```python
from build123d import *

# Parameters (mm, degrees)
F0_R     = 57
F1_DEPTH = 5
F0_W     = 15
F0_H     = 15
F2_DEPTH = 20
F3_SIZE  = 5


with BuildPart() as f1:
    # F0 (on Top) → F1 (new body)
    with BuildSketch(Plane.XY):
        Polygon((-45, -60), (45, -60), (45, -45), (60, -45), (60, 45), (45, 45), (45, 60), (-45, 60), (-45, 45), (-60, 45), (-60, -45), (-45, -45), align=None)
        Circle(F0_R, mode=Mode.SUBTRACT)
    extrude(amount=F1_DEPTH)

    # F0 (on Top) → F2 (join)
    with BuildSketch(Plane.XY):
        with Locations((-52.5, 52.5)):
            Rectangle(F0_W, F0_H)
        with Locations((52.5, 52.5)):
            Rectangle(F0_W, F0_H)
        with Locations((52.5, -52.5)):
            Rectangle(F0_W, F0_H)
        with Locations((-52.5, -52.5)):
            Rectangle(F0_W, F0_H)
    extrude(amount=F2_DEPTH)

    # F3
    f3_edges = [f1.edges().sort_by_distance(p)[0] for p in [
        (-60, -45, 12.5),
        (-45, -60, 12.5),
        (45, -60, 12.5),
        (60, -45, 12.5),
        (45, 60, 12.5),
        (60, 45, 12.5),
        (-60, 45, 12.5),
        (-45, 60, 12.5),
    ]]
    chamfer(f3_edges, length=F3_SIZE)


solid = f1.part
```
CAD build for the part. Positions are in the model's coordinates, mm. A direction names the side the tool comes from. Coordinates: 2 decimals unless noted, no trailing zeros. Write each loop counter-clockwise with the first axis right and the second up, starting at its lowest first coordinate (ties: lowest second). Pieces come first, ordered by that corner, then holes. Notation, with made-up numbers: (83, 58) -> (118, 58) arc R9 cw to (118, 66) -> close; hole circle Ø3 at (40.25, -34.5). An arc over 180 degrees is marked (long way). Use CSV: the item, a comma, the result in double quotes. Start each with the question number.
Item 1: Two-plate mould, pull along X, no slides. Class faces 1 (the flat face through (-48, -58, 12)), 2 (the flat face through (-50, 45, 12)), 3 (the flat face through (48, -58, 12)), 4 (the flat face through (-57, 47, 12)): +X half, -X half, draft (parallel to the pull), parting line (faces both ways), or undercut.
Item 2: Band-saw the part on A-A, the plane x = 0. Write the cut outline in (y, z), plus the area to 3 significant figures.
Item 3: Wall check: probe 1 along Y at (x, z) = (0, 2.6); probe 2 along Y at (x, z) = (-50.5, 7.5); probe 3 along Z at (x, y) = (-48.5, 42). Give the ranges that are in metal, low to high.
Item 4: Band-saw the part on C-C, the plane z = 2.25. Write the cut outline in (x, y).
Item 5: Tool access for faces 5 (the flat face through (-60, -1, 3)), 6 (the flat face through (-50, -45, 12)), 7 (the flat face through (-45, -50, 12)), 8 (the flat face through (48, 58, 12)), 9 (the flat face through (-36, 45, 0)): list every direction of +Z, -Z, +X, -X, +Y, -Y with a clear straight run to the whole face (end or side of a thin tool).
Item 6: Band-saw the part on D-D, the plane z = 14.5. Write the cut outline in (x, y), plus the area to 3 significant figures.
Response values:
1,face 1,"undercut"
1,face 2,"draft"
1,face 3,"undercut"
1,face 4,"-X half"
2,outline,"(-60, 0) -> (-57, 0) -> (-57, 5) -> (-60, 5) -> close; (57, 0) -> (60, 0) -> (60, 5) -> (57, 5) -> close"
2,area,"30.0 mm2"
3,probe 1,"y = -60 to -57, 57 to 60"
3,probe 2,"y = -60 to -45, 45 to 60"
3,probe 3,"z = 0 to 5"
4,outline,"(-60, -60) -> (60, -60) -> (60, 60) -> (-60, 60) -> close; hole circle Ø114 at (0, 0)"
5,face 5,"+Z, -Z, -X, +Y, -Y"
5,face 6,"+Z, +X, -X"
5,face 7,"+Z, +Y, -Y"
5,face 8,"+Z, +Y"
5,face 9,"-Z, +X, -X, +Y, -Y"
6,outline,"(-60, -60) -> (-50, -60) -> (-45, -55) -> (-45, -45) -> (-55, -45) -> (-60, -50) -> close; (-60, 50) -> (-55, 45) -> (-45, 45) -> (-45, 55) -> (-50, 60) -> (-60, 60) -> close; (45, -55) -> (50, -60) -> (60, -60) -> (60, -50) -> (55, -45) -> (45, -45) -> close; (45, 45) -> (55, 45) -> (60, 50) -> (60, 60) -> (50, 60) -> (45, 55) -> close"
6,area,"800 mm2"
